Check sheet for the modelled part. Datum: model origin and axes. Units: mm. A direction names the side the tool comes from. Round coordinates to 2 decimals unless told otherwise and drop trailing zeros. Order: outer loops, then holes, each group sorted by start corner. A loop starts at its lowest first (then second) coordinate and runs counter-clockwise, first axis right, second up. Notation, with made-up numbers: (88.5, -13.75) -> (93.5, -13.75) arc R24 ccw to (93.5, 23.25) -> close; hole circle Ø7 at (53, 70). An arc over 180 degrees is marked (long way). Answer in a Markdown table with one row per item.
from build123d import *

# Parameters (mm, degrees)
F0_R     = 17.5
F1_DEPTH = 30
F2_R     = 19
F3_DEPTH = 2
F4_SIZE  = 1
F5_SIZE  = 1


with BuildPart() as f1:
    # F0 (on Top) → F1 (new body)
    with BuildSketch(Plane.XY):
        Circle(F0_R)
        with BuildLine():
            ThreePointArc((-15.627753, -4.453744), (-13.778547, 8.614764), (-2.839454, 16))
            Line((-2.839454, 16), (2.839454, 16))
            ThreePointArc((2.839454, 16), (13.778547, 8.614764), (15.627753, -4.453744))
            Line((15.627753, -4.453744), (13.140933, -9.559204))
            ThreePointArc((13.140933, -9.559204), (0, -16.25), (-13.140933, -9.559204))
            Line((-13.140933, -9.559204), (-15.627753, -4.453744))
        make_face(mode=Mode.SUBTRACT)
    extrude(amount=F1_DEPTH)

    # F2 (on face) → F3 (join)
    with BuildSketch(Plane(origin=(0, 0, 0), x_dir=(1, 0, 0), z_dir=(0, 0, -1))):
        Circle(F2_R)
        with BuildLine():
            Line((-15.627753, 4.453744), (-13.140933, 9.559204))
            ThreePointArc((-13.140933, 9.559204), (0, 16.25), (13.140933, 9.559204))
            Line((13.140933, 9.559204), (15.627753, 4.453744))
            ThreePointArc((15.627753, 4.453744), (13.778547, -8.614764), (2.839454, -16))
            Line((2.839454, -16), (-2.839454, -16))
            ThreePointArc((-2.839454, -16), (-13.778547, -8.614764), (-15.627753, 4.453744))
        make_face(mode=Mode.SUBTRACT)
    extrude(amount=F3_DEPTH)

    # F4
    f4_edges = [f1.edges().sort_by_distance(p)[0] for p in [
        (-17.5, 0, 30),
    ]]
    chamfer(f4_edges, length=F4_SIZE)

    # F5
    f5_edges = [f1.edges().sort_by_distance(p)[0] for p in [
        (0, -16.25, -2),
        (14.384343, -7.006474, -2),
        (13.778547, 8.614764, -2),
        (0, 16, -2),
        (-13.778547, 8.614764, -2),
        (-14.384343, -7.006474, -2),
    ]]
    chamfer(f5_edges, length=F5_SIZE)


solid = f1.part
Item 1: Cross-section at A-A (x = 0). Record the boundary of the cut face in (y, z).
Result sheet:
| item | result |
|---|---|
| outline | (-19, -2) -> (-17.25, -2) -> (-16.25, -1) -> (-16.25, 30) -> (-16.5, 30) -> (-17.5, 29) -> (-17.5, 0) -> (-19, 0) -> close; (16, -1) -> (17, -2) -> (19, -2) -> (19, 0) -> (17.5, 0) -> (17.5, 29) -> (16.5, 30) -> (16, 30) -> close |
Item 2: Mould release check, pull along Y, two halves, no side actions. Record for faces 1 (the flat face through (-14.86, -7.19, -1.51)), 2 (the flat face through (-4, 17, -2)), 3 (the cylindrical face through (-13.887, -10.648, 14.297)): pulls with the +Y half, pulls with the -Y half, needs draft (parallel to the pull), parting line crosses it, or undercut.
Result sheet:
| item | result |
|---|---|
| face 1 | undercut |
| face 2 | needs draft |
| face 3 | parting line crosses it |
Item 3: Cross-section at B-B (z = 14.5). Record the boundary of the cut face in (x, y).
Result sheet:
| item | result |
|---|---|
| outline | circle Ø35 at (0, 0); hole (-15.63, -4.45) -> (-13.14, -9.56) arc R16.25 ccw to (13.14, -9.56) -> (15.63, -4.45) arc R16.25 ccw to (2.84, 16) -> (-2.84, 16) arc R16.25 ccw to start |
Item 4: Set-up check for faces 4 (the flat face through (6, 17, 0)), 5 (the flat face through (14.8, -7.3, -1.5)), 6 (the flat face through (14.37, -7.04, 14.72)): record each of +Z, -Z, +X, -X, +Y, -Y from which the full face is reachable in a straight line by a thin tool's end or side.
Result sheet:
| item | result |
|---|---|
| face 4 | +Z |
| face 5 | -Z |
| face 6 | +Z, -Z |
Item 5: Depth check by flat-ended pin: P1, Ø1.5, axis at x = 8, z = 14, coming from the -Y side; P2, Ø8, axis at x = -0.5, z = 14, coming from the +Y side; P3, Ø1.5, axis at y = -9, z = 24, coming from the +X side. Enter the tip coordinate at first touch or a pass-through.
Result sheet:
| item | result |
|---|---|
| P1 | stops at y = -15.93 |
| P2 | stops at y = 17.5 |
| P3 | stops at x = 15.43 |
Item 6: Scan lines: line 1 (Y direction, x = -8.5, z = 1); line 2 (X direction, y = -10.5, z = 1); line 3 (Y direction, x = -5, z = 28). Record each from-to range of solid material in increasing order. Write a range as [from, to].
Result sheet:
| item | result |
|---|---|
| line 1 | y = [-15.3, -13.85], [13.85, 15.3] |
| line 2 | x = [-14, -12.4], [12.4, 14] |
| line 3 | y = [-16.77, -15.46], [15.46, 16.77] |
